Can you work these out from the model? Positions are in its coordinate system, mm. Face numbers are marked on the shaded views. A direction names the side the tool comes from. Round coordinates to 2 decimals unless told otherwise and drop trailing zeros. Order: outer loops, then holes, each group sorted by start corner. A loop starts at its lowest first (then second) coordinate and runs counter-clockwise, first axis right, second up.
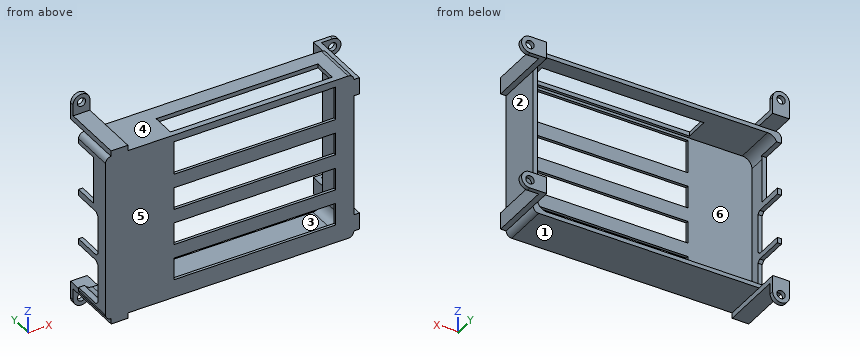
Autodesk Inventor part; units mm, degrees
ref_plane "Work Plane1" through (-2, 0, -30) normal (0, 0, 1) x (1, 0, 0)
ref_plane "YZ Plane" through (0, 0, 0) normal (1, 0, 0) x (0, 1, 0)
ref_plane "XZ Plane" through (0, 0, 0) normal (0, 1, 0) x (-1, 0, 0)
sketch "Sketch1" plane through (0, 0, 0) normal (0, 1, 0) x (-1, 0, 0)
  line L0 (2, 0) -> (87, 0)
  line L1 (89, -2) -> (89, -58)
  line L2 (87, -60) -> (2, -60)
  line L3 (0, -58) -> (0, -2)
  arc A0 (2, 0) -> (0, -2) centre (2, -2) ccw
  arc A1 (0, -58) -> (2, -60) centre (2, -58) ccw
  arc A2 (87, -60) -> (89, -58) centre (87, -58) ccw
  arc A3 (89, -2) -> (87, 0) centre (87, -2) ccw
  point P0 (0, 0)
  point P1 (89, -60)
  point P2 (0, -60)
  dimension "d0" = 60
  dimension "d1" = 89
  dimension "d2" = 2
extrude "Extrusion1" add sketch "Sketch1" along normal blind 1
sketch "Sketch2" plane through (0, 1, 0) normal (0, 1, 0) x (1, 0, 0)
  line L0 (-87, 0) -> (-2, 0)
  line L1 (0, 2) -> (0, 58)
  line L2 (-2, 60) -> (-87, 60)
  line L3 (-89, 58) -> (-89, 2)
  line L4 (-89, 58) -> (-89, 2)
  line L5 (-87, 0) -> (-2, 0)
  line L6 (0, 2) -> (0, 58)
  line L7 (-2, 60) -> (-87, 60)
  arc A0 (-89, 2) -> (-87, 0) centre (-87, 2) ccw
  arc A1 (-87, 60) -> (-89, 58) centre (-87, 58) ccw
  arc A2 (0, 58) -> (-2, 60) centre (-2, 58) ccw
  arc A3 (-2, 0) -> (0, 2) centre (-2, 2) ccw
  line L8 (-84, 1.5) -> (-5, 1.5)
  line L9 (-1.5, 5) -> (-1.5, 55)
  line L10 (-5, 58.5) -> (-84, 58.5)
  line L11 (-87.5, 55) -> (-87.5, 5)
  arc A4 (-5, 1.5) -> (-1.5, 5) centre (-5, 5) ccw
  arc A5 (-1.5, 55) -> (-5, 58.5) centre (-5, 55) ccw
  arc A6 (-84, 58.5) -> (-87.5, 55) centre (-84, 55) ccw
  arc A7 (-87.5, 5) -> (-84, 1.5) centre (-84, 5) ccw
  point P0 (0, 0)
  dimension "d5" = 2
  dimension "d6" = 1.5
  dimension "d7" = 1.5
  dimension "d8" = 1.5
  dimension "d9" = 1.5
  dimension "d10" = 3.5
extrude "Extrusion2" add sketch "Sketch2" along normal blind 15
sketch "Sketch3" plane through (-87, 0, 0) normal (0, 0, 1) x (1, 0, 0)
  line L0 (22.5, 10.5) -> (80.5, 10.5)
  line L1 (80.5, 10.5) -> (80.5, 2)
  line L2 (80.5, 2) -> (22.5, 2)
  line L3 (22.5, 2) -> (22.5, 10.5)
  line L4 (87, 0) -> (87, 16)
  line L5 (0, 0) -> (85, 0)
  dimension "d13" = 58
  dimension "d14" = 8.5
  dimension "d15" = 6.5
  dimension "d16" = 2
extrude "Extrusion3" cut sketch "Sketch3" against normal up to surface (1.5 mm away)
sketch "Sketch4" plane through (0, 1, 0) normal (0, 1, 0) x (1, 0, 0)
  line L0 (-64.5, 1.5) -> (-6.5, 1.5)
  line L1 (-64.5, 2.5) -> (-6.5, 2.5)
  line L2 (-6.5, 2.5) -> (-6.5, 14.5)
  line L3 (-6.5, 14.5) -> (-64.5, 14.5)
  line L4 (-64.5, 14.5) -> (-64.5, 2.5)
  line L5 (-6.5, 1.5) -> (-6.5, 2.5) construction
  point P0 (0, 0)
  dimension "d19" = 12
  dimension "d20" = 58
  dimension "d21" = 1
extrude "Extrusion4" cut sketch "Sketch4" against normal up to surface (1 mm away)
sketch "Sketch5" plane through (0, 1, 0) normal (0, 1, 0) x (1, 0, 0)
  line L0 (-64.5, 19.5) -> (-6.5, 19.5)
  line L1 (-6.5, 19.5) -> (-6.5, 27.5)
  line L2 (-6.5, 27.5) -> (-64.5, 27.5)
  line L3 (-64.5, 27.5) -> (-64.5, 19.5)
  line L4 (-64.5, 2.5) -> (-64.5, 14.5)
  line L5 (-64.5, 14.5) -> (-6.5, 14.5)
  line L6 (-64.5, 32.5) -> (-6.5, 32.5)
  line L7 (-6.5, 32.5) -> (-6.5, 40.5)
  line L8 (-6.5, 40.5) -> (-64.5, 40.5)
  line L9 (-64.5, 40.5) -> (-64.5, 32.5)
  line L10 (-64.5, 45.5) -> (-6.5, 45.5)
  line L11 (-6.5, 45.5) -> (-6.5, 53.5)
  line L12 (-6.5, 53.5) -> (-64.5, 53.5)
  line L13 (-64.5, 53.5) -> (-64.5, 45.5)
  point P0 (0, 0)
  dimension "d24" = 8
  dimension "d25" = 58
  dimension "d26" = 5
  dimension "d27" = 5
  dimension "d28" = 8
  dimension "d29" = 58
  dimension "d30" = 5
  dimension "d31" = 8
extrude "Extrusion5" cut sketch "Sketch5" against normal up to surface (1 mm away)
sketch "Sketch6" plane through (-89, 0, -58) normal (-1, 0, 0) x (0, 0, 1)
  line L0 (54.25, 7) -> (37.25, 7)
  line L1 (37.25, 7) -> (37.25, 16)
  line L2 (37.25, 16) -> (54.25, 16)
  line L3 (54.25, 16) -> (54.25, 7)
  line L4 (0, 0) -> (56, 0)
  line L5 (0, 16) -> (56, 16)
  line L6 (58, 0) -> (58, 16)
  dimension "d34" = 7
  dimension "d35" = 3.75
  dimension "d36" = 17
extrude "Extrusion6" cut sketch "Sketch6" against normal blind 2
sketch "Sketch7" plane through (-89, 0, -58) normal (-1, 0, 0) x (0, 0, 1)
  line L0 (35, 16) -> (19, 16)
  line L1 (19, 16) -> (19, 5.6)
  line L2 (19, 5.6) -> (20, 4.6)
  line L3 (20, 4.6) -> (34, 4.6)
  line L4 (34, 4.6) -> (35, 5.6)
  line L5 (35, 5.6) -> (35, 16)
  line L6 (37.25, 7) -> (37.25, 16)
  line L7 (0, 16) -> (37.25, 16)
  line L8 (0, 0) -> (56, 0)
  line L9 (2, 4.6) -> (16, 4.6)
  line L10 (16, 4.6) -> (17, 5.6)
  line L11 (17, 5.6) -> (17, 16)
  line L12 (17, 16) -> (1, 16)
  line L13 (1, 16) -> (1, 5.6)
  line L14 (1, 5.6) -> (2, 4.6)
  point P0 (58, 0)
  point P1 (17, 16)
  point P2 (1, 16)
  dimension "d39" = 2.25
  dimension "d40" = 14
  dimension "d41" = 16
  dimension "d42" = 4.6
  dimension "d45" = 18
extrude "Extrusion7" cut sketch "Sketch7" against normal blind 2.5
sketch "Sketch8" plane through (0, 0, 0) normal (0, -1, 0) x (1, 0, 0)
  line L0 (0, -2) -> (0, -58)
  line L1 (0, -2) -> (2, -2)
  line L2 (2, -2) -> (2, -8)
  line L3 (2, -8) -> (0, -8)
  line L4 (0, -8) -> (0, -2)
  line L5 (-87, 0) -> (-2, 0)
  line L6 (-87, 0) -> (-81, 0)
  line L7 (-81, 0) -> (-81, 2)
  line L8 (-81, 2) -> (-87, 2)
  line L9 (-87, 2) -> (-87, 0)
  point P0 (0, 0)
  dimension "d52" = 6
  dimension "d53" = 2
  dimension "d54" = 6
  dimension "d55" = 2
extrude "Extrusion8" add sketch "Sketch8" against normal blind 24
sketch "Sketch9" plane through (0, 24, 0) normal (0, 1, 0) x (1, 0, 0)
  arc A0 (-89, 2) -> (-87, 0) centre (-87, 2) ccw
  line L0 (-87, 0) -> (-81, 0)
  line L1 (-81, 0) -> (-81, -6)
  line L2 (-81, -6) -> (-87, -6)
  line L3 (-87, -6) -> (-87, 0)
  circle A1 centre (-84, -6) radius 3
  circle A2 centre (-84, -6) radius 1.5
  line L4 (2, 8) -> (0, 8)
  line L5 (0, 8) -> (6, 8)
  line L6 (6, 8) -> (6, 2)
  line L7 (6, 2) -> (0, 2)
  line L8 (0, 2) -> (0, 8)
  circle A3 centre (6, 5) radius 3
  circle A4 centre (6, 5) radius 1.5
  point P0 (0, 0)
  point P1 (6, 2)
  dimension "d58" = 6
  dimension "d59" = 6
  dimension "d60" = 3
  dimension "d61" = 6
  dimension "d62" = 6
  dimension "d63" = 3
extrude "Extrusion9" add sketch "Sketch9" against normal blind 1.5 contours L0 L1 A1 L3 | A1 L2 A2 | L2 A2 A1 | L5 A3 L7 L8 L4 | A3 L6 A4 | L6 A4 A3
ref_plane "Work Plane1" through (-2, 0, -30) normal (0, 0, 1) x (1, 0, 0)
mirror "Mirror1" about plane through (-2, 0, -30) normal (0, 0, 1) of "Extrusion9", "Extrusion8"
properties part number "raspi_cover"
(1) If we mould it in two halves opening along X, with no side actions, what happens to the marked faces 1, 2 and 3? For each: pulls with the +X half, pulls with the -X half, needs draft (parallel to the pull), parting line crosses it, or undercut.
(2) I want a section at B-B, the plane z = -9.5. List the corners of the cut face in (x, y) for me, plus the area to 3 significant figures.
(3) Please list where these lines run through material, in increasing order: probe 1 along Z at (x, y) = (6, 23.1); probe 2 along Z at (x, y) = (-84, 23.25); probe 3 along Z at (x, y) = (-13, 14.25).
(4) I want a section at C-C, the plane y = 17.75. List the corners of the cut face in (x, z) for me.
(5) On a 3-axis mill with a long thin cutter (end or side, diameter ignored), from which of +Z, -Z, +X, -X, +Y, -Y can I reach the whole of each face in a straight line? I mean the marked faces 4, 5 and 6. Say none if no direction works.
(6) I want a section at A-A, the plane x = -31. List the corners of the cut face in (y, z) for me, plus the area to 4 significant figures.
(7) I'm going to push flat-ended pins straight in: pin 1 Ø5 at (x, y) = (4, 7) entering from -Z; pin 2 Ø1.5 at (y, z) = (8, -60) entering from -X; pin 3 Ø4 at (y, z) = (13.5, -60.5) entering from -X. Where does each tip first touch, or does it pass through?
Ans:
1. face 1: needs draft
1. face 2: pulls with the +X half
1. face 3: undercut
2. outline: (-89, 0) - (-64.5, 0) - (-64.5, 1) - (-87.5, 1) - (-87.5, 7) - (-89, 7) - close; (-6.5, 0) - (0, 0) - (0, 16) - (-1.5, 16) - (-1.5, 1) - (-6.5, 1) - close
2. area: 62.5 mm2
3. probe 1: z = -58 to -56.5, -53.5 to -52, -8 to -6.5, -3.5 to -2
3. probe 2: z = -69 to -67.5, -64.5 to -60, 0 to 4.5, 7.5 to 9
3. probe 3: z = -60 to -58.5, -1.5 to 0
4. outline: (-87, -62) - (-81, -62) - (-81, -60) - (-87, -60) - close; (-87, 0) - (-81, 0) - (-81, 2) - (-87, 2) - close; (0, -58) - (2, -58) - (2, -52) - (0, -52) - close; (0, -8) - (2, -8) - (2, -2) - (0, -2) - close
5. face 4: +Z, +X, +Y, -Y
5. face 5: +Z, -Z, +X, -X, -Y
5. face 6: +Y
6. outline: (0, -60) - (16, -60) - (16, -58.5) - (1, -58.5) - (1, -53.5) - (0, -53.5) - close; (0, -45.5) - (1, -45.5) - (1, -40.5) - (0, -40.5) - close; (0, -32.5) - (1, -32.5) - (1, -27.5) - (0, -27.5) - close; (0, -19.5) - (1, -19.5) - (1, -14.5) - (0, -14.5) - close; (0, -2.5) - (1, -2.5) - (1, -1.5) - (2, -1.5) - (2, 0) - (0, 0) - close; (10.5, -1.5) - (16, -1.5) - (16, 0) - (10.5, 0) - close
6. area: 56.25 mm2
7. pin 1: stops at z = -58
7. pin 2: stops at x = -88.56
7. pin 3: stops at x = -88.94
